Autodesk Inventor part; units mm, degrees
ref_plane "YZ Plane" through (0, 0, 0) normal (1, 0, 0) x (0, 1, 0)
ref_plane "XZ Plane" through (0, 0, 0) normal (0, 1, 0) x (-1, 0, 0)
ref_plane "XY Plane" through (0, 0, 0) normal (0, 0, 1) x (1, 0, 0)
sketch "Sketch1" plane through (0, 0, 0) normal (0, 0, 1) x (1, 0, 0)
  line L0 (0, 0) -> (0, -2.7)
  line L1 (0, -2.7) -> (-2.5, -2.7)
  line L2 (-2.5, -2.7) -> (-2.5, 25.3)
  line L3 (0, 25.3) -> (-2.5, 25.3)
  line L4 (0, 25.3) -> (0, 22.6)
  line L5 (0, 22.6) -> (2, 22.6)
  line L6 (2, 27.3) -> (2, 22.6)
  line L7 (-4.5, 27.3) -> (2, 27.3)
  line L8 (-4.5, -4.7) -> (-4.5, 27.3)
  line L9 (-4.5, -4.7) -> (2, -4.7)
  line L10 (2, 0) -> (2, -4.7)
  line L11 (0, 0) -> (2, 0)
  line L12 (-0.2, 25.1) -> (-2.3, 25.1)
  line L13 (-2.3, 25.1) -> (-2.3, -2.5)
  line L14 (-2.3, -2.5) -> (-0.2, -2.5)
  line L15 (-0.2, -2.5) -> (-0.2, 25.1)
  line L16 (0, 22.6) -> (0, 22.4) construction
  line L17 (1, 13) -> (2, 13)
  line L18 (1, 9.6) -> (1, 13)
  line L19 (2, 9.6) -> (1, 9.6)
  line L20 (2, 13) -> (2, 9.6)
  line L21 (1, 11.3) -> (1.2, 11.3) construction
  line L22 (2, 13) -> (1.2, 13)
  line L23 (1.2, 13) -> (1.2, 9.6)
  line L24 (1.2, 9.6) -> (2, 9.6)
  line L25 (2, 9.6) -> (2, 13)
  line L26 (1.2, 13) -> (1.2, 13.2)
  line L27 (2, 13.2) -> (-0.2, 13.2)
  line L28 (-0.2, 13.2) -> (-0.2, 22.4)
  line L29 (-0.2, 22.4) -> (2, 22.4)
  line L30 (2, 22.4) -> (2, 13.2)
  line L31 (2, 13.2) -> (2, 13)
  line L32 (2, 9.6) -> (1.2, 9.6)
  line L33 (1.2, 9.6) -> (1.2, 9.4)
  line L34 (1.2, 9.4) -> (2, 9.4)
  line L35 (2, 9.4) -> (2, 9.6)
  line L36 (2, 9.4) -> (-0.2, 9.4)
  line L37 (-0.2, 9.4) -> (-0.2, 0.2)
  line L38 (-0.2, 0.2) -> (2, 0.2)
  line L39 (2, 0.2) -> (2, 9.4)
  point P0 (-1.25, 11.3)
  point P1 (-1.25, 11.3)
  dimension "d0" = 2.1
  dimension "d1" = 27.6
  dimension "d2" = 0.2
  dimension "d3" = 0.2
  dimension "d4" = 0.2
  dimension "d5" = 0.2
  dimension "d6" = 9.2
extrude "Extrusion1" add sketch "Sketch1" against normal blind 2 contours L15 L14 L13 L12 | L29 L30 L27 L15 | L36 L34 L39 L38 L15 | L27 L31 L17 L26 | L33 L19 L35 L34 | L17 L20 L19 L23
sketch "Sketch2" plane through (2, 0.2, 0) normal (1, 0, 0) x (0, 0, -1)
  arc A0 (9, -0.2) -> (9, 9.4) centre (9, 4.6) ccw
  arc A1 (9, 12.8) -> (9, 22.4) centre (9, 17.6) ccw
  circle A2 centre (9, 4.6) radius 4.6
  circle A3 centre (9, 17.6) radius 4.6
  line L0 (2, 22.2) -> (2, 0)
  line L1 (9, 0) -> (2, 0)
  line L2 (9, 9.2) -> (2, 9.2)
  line L3 (2, 0) -> (2, 9.2)
  line L4 (9, 13) -> (2, 13)
  line L5 (2, 13) -> (2, 22.2)
  line L6 (0, 22.2) -> (2, 22.2)
  line L7 (9, 22.2) -> (2, 22.2)
  point P0 (0, -0.2)
  dimension "d12" = 9.2
  dimension "d13" = 9.2
extrude "Extrusion3" add sketch "Sketch2" against normal blind 2 contours L0 L7 A3 L4 | A2 L1 L0 L2
properties part number "prototype7_2_3DPrint"
Check sheet for the modelled part. Datum: model origin and axes. Units: mm. A direction names the side the tool comes from. Round coordinates to 2 decimals unless told otherwise and drop trailing zeros. Order: outer loops, then holes, each group sorted by start corner. A loop starts at its lowest first (then second) coordinate and runs counter-clockwise, first axis right, second up. Notation, with made-up numbers: (63, -17) - (68, -17) arc R20 ccw to (68, -4) - close; hole circle Ø9 at (86.5, 74.25). An arc over 180 degrees is marked (long way). Write item = value, one per line.
Q1. Section check A-A (x = 0.9). Record the boundary of the cut face in (y, z), and give its area (3 significant figures).
Computed:
outline = (0.2, -9) arc R4.6 cw to (9.4, -9) - (9.4, 0) - (0.2, 0) - close; (13.2, -9) arc R4.6 cw to (22.4, -9) - (22.4, 0) - (13.2, 0) - close
area = 99.1 mm^2
Q2. Section check B-B (z = -4). Record the boundary of the cut face in (x, y).
Computed:
outline = (0, 0.2) - (2, 0.2) - (2, 9.4) - (0, 9.4) - close; (0, 13.2) - (2, 13.2) - (2, 22.4) - (0, 22.4) - close
Q3. Section check C-C (y = 4.8). Record the boundary of the cut face in (x, z).
Computed:
outline = (-2.3, -2) - (0, -2) - (0, -4.4) - (2, -4.4) - (2, 0) - (-2.3, 0) - close
Q4. Go/stop test with flat-tipped pins: pin 1 (1.1 mm diameter, centred on x = 0.5, z = -3.5, fed in from +Y); pin 2 (1.1 mm diameter, centred on x = 0.5, z = -2.5, fed in from -Y); pin 3 (0.7 mm diameter, centred on x = -1, y = 12, fed in from -Z); pin 4 (1 mm diameter, centred on y = 12, z = -6, fed in from +X). Record where each tip stops, or that it passes through.
Computed:
pin_1 = 22.4
pin_2 = 0.2
pin_3 = -2
pin_4 = through
Q5. Tool access check on faces 1 (the face through (-0.2, -1, -1)), 2 (the face through (-0.2, 24, -1)), 3 (the face through (1.2, 11, -1)). Record the directions out of +Z, -Z, +X, -X, +Y, -Y that give a thin tool (end or side, any length) a straight path to the whole face; none if there is none.
Computed:
face_1 = +Z, -Z, +X, -Y
face_2 = +Z, -Z, +X, +Y
face_3 = +Z, -Z
Q6. Section check D-D (z = -6). Record the boundary of the cut face in (x, y), and give its area (3 significant figures).
Computed:
outline = (0, 0.2) - (2, 0.2) - (2, 1.31) - (0, 1.31) - close; (0, 8.29) - (2, 8.29) - (2, 9.4) - (0, 9.4) - close; (0, 13.2) - (2, 13.2) - (2, 14.31) - (0, 14.31) - close; (0, 21.29) - (2, 21.29) - (2, 22.4) - (0, 22.4) - close
area = 8.90 mm^2
Q7. Draft check along Y on faces 4 (the face through (2, 11, -1)), 5 (the face through (1, 9.4, -4)), 6 (the face through (-1, -2.5, -1)). Enter one of: pulls with the +Y half, pulls with the -Y half, needs draft (parallel to the pull), parting line crosses it, or undercut.
Computed:
face_4 = needs draft
face_5 = undercut
face_6 = pulls with the -Y half
Q8. Thickness scan on line 1 along Y through (x, z) = (1.4, -3.75); line 2 along Y through (x, z) = (0.45, -6.75); line 3 along Y through (x, z) = (1.4, -5.75). Record the ranges inside material, lowest first.
Computed:
line_1 = 0.2 to 9.4, 13.2 to 22.4
line_2 = 0.2 to 0.79, 8.81 to 9.4, 13.2 to 13.79, 21.81 to 22.4
line_3 = 0.2 to 1.54, 8.06 to 9.4, 13.2 to 14.54, 21.06 to 22.4
